Can you work these out from the drawing? Everything is in mm from the part's minimum corner. A direction names the side the tool comes from. Give positions to 0.01 mm unless a question says otherwise; leave off trailing zeros. Loops run counter-clockwise (first coordinate to the right, second up) from the corner with the lowest first, then second, coordinate; pieces in that order, holes last.
Q1. If we section it at A-A (z = 1.7): Please give me the cut outline in (x, y).
Q2. I need wall thicknesses on line 1 (Y direction, x = 8, z = 1.85); line 2 (X direction, y = 4.25, z = 1.35). Which ranges of each line are inside material? Lowest first, please.
Q3. Will these pins go through, and if not, where does the flat tip stop? P1, Ø2.5, axis at x = 10, y = 5, coming from the -Z side; P2, Ø1.6, axis at y = 2.5, z = 3, coming from the +X side; P3, Ø2.5, axis at x = 5, z = 2, coming from the -Y side; P4, Ø2, axis at y = 3, z = 3.5, coming from the -X side.
Q4. For the marked faces 1, 2 and 3, which set-ups out of +Z, -Z, +X, -X, +Y, -Y let a thin tool reach every point of the face, with its end or its side?
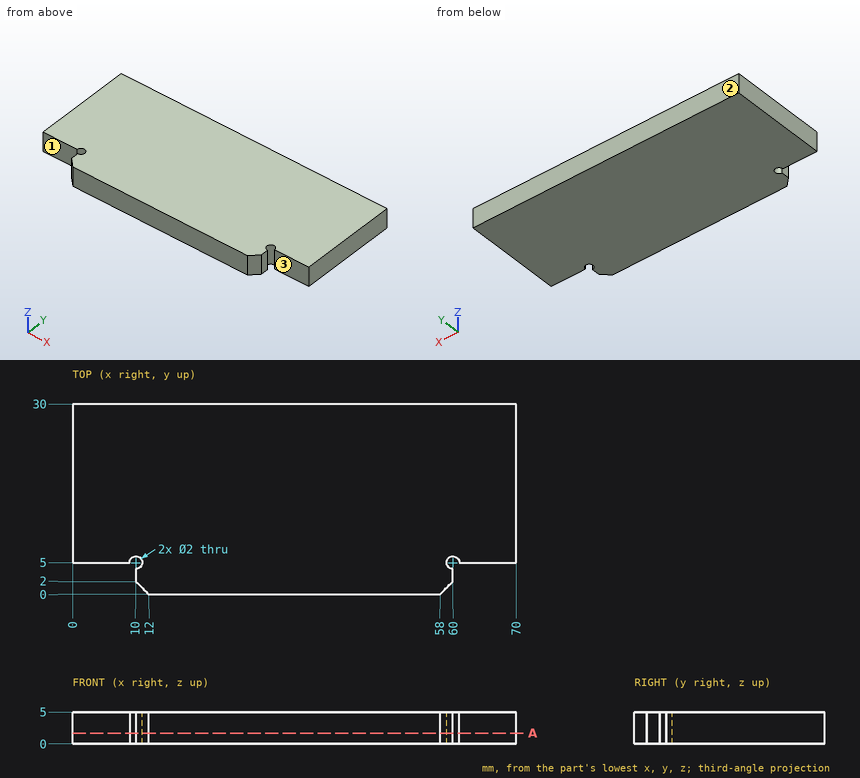
Check sheet entries:
1. outline: (0, 5) - (9, 5) arc R1 cw (long way) to (10, 4) - (10, 2) - (12, 0) - (58, 0) - (60, 2) - (60, 4) arc R1 cw (long way) to (61, 5) - (70, 5) - (70, 30) - (0, 30) - close
2. line 1: y = 5 to 30
2. line 2: x = 10.66 to 59.34
3. P1: stops at z = 0
3. P2: stops at x = 60
3. P3: stops at y = 5
3. P4: stops at x = 10
4. face 1: +Z, -Z, -X, -Y
4. face 2: +Z, -Z, +X, -X, +Y
4. face 3: +Z, -Z, +X, -Y
